Design review of the part built by this model. Coordinates are the model's own, in mm. A direction names the side the tool comes from. Coordinates: 2 decimals unless noted, no trailing zeros. Loops run counter-clockwise (first coordinate to the right, second up) from the corner with the lowest first, then second, coordinate; pieces in that order, holes last. Notation, with made-up numbers: (28, 26.25) -> (63, 26.25) arc R18 ccw to (63, 43.25) -> close; hole circle Ø3 at (39.25, -2.75). An arc over 180 degrees is marked (long way). Use a Markdown table: item, result. Add a question column.
Q1. Take a section at B-B on y = 20. Write out the cut boundary in (x, z), plus the area to 3 significant figures.
Q2. For faces 4 (the face through (-5.37, 0.99, 1.19)), 5 (the face through (7.3, -20, 0)), 6 (the face through (0, 80, 0)), 7 (the face through (5.38, 28.68, -8.43)), 8 (the face through (10, 20, 4.6)), list the 3-axis set-ups (+Z, -Z, +X, -X, +Y, -Y) from which the entire face can be reached by the end or side of a thin tool; tool diameter is ignored.
Q3. Take a section at A-A on y = -6.5. Write out the cut boundary in (x, z), plus the area to 3 significant figures.
Q4. Draft analysis for pull direction Z (two halves, no side actions). For faces 1 (the face through (5.684, 70.103, -1.79)), 2 (the face through (0.8, 8, 10.2)), 3 (the face through (3.64, 70.07, -1.15)), state which applies: pulls with the +Z half, pulls with the -Z half, needs draft (parallel to the pull), parting line crosses it, or undercut.
Q5. For probe 1 along X at (y, z) = (1.55, 0); probe 2 along X at (y, z) = (47, -0.5); probe 3 along Z at (x, y) = (0, 44.5), list the stretches that pass through material, from the lowest coordinate up.
Q6. Clearance check with flat-ended pins moving along their axes: pin 1 Ø12 at (x, z) = (0, 0) entering from -Y; pin 2 Ø10 at (x, y) = (7, 36.5) entering from +Z; pin 3 Ø3.5 at (x, z) = (4.5, 10) entering from +Y. State where each tip first meets the part, or that it passes through.
from build123d import *

# Parameters (mm, degrees)
SKETCH1_R               = 12
BOSS_EXTRUDE1_DEPTH     = 55
SKETCH2_R               = 2
SKETCH3_R               = 9
SKETCH3_R_2             = 7
BOSS_EXTRUDE2_DEPTH     = 20
SKETCH5_R               = 5.5
CUT_EXTRUDE2_DEPTH      = 4
SKETCH6_W               = 20
SKETCH6_H               = 25
CUT_EXTRUDE3_DEPTH      = 3
CUT_EXTRUDE4_DEPTH      = 85.380092576
CUT_EXTRUDE4_DEPTH_BACK = 85.380092576
SKETCH7_W               = 7.4
SKETCH7_H               = 25
FILLET1_R               = 1.5


# Read off the part's stored shape, not the designer's step: Shell1
with BuildPart() as part:
    # Sketch1 → Boss-Extrude1 (new body)
    with BuildSketch(Plane(origin=(0, 0, 0), x_dir=(1, 0, 0), z_dir=(0, 1, 0))):
        with Locations(Location((0, 0, 0), (0, 0, 270))):
            Circle(SKETCH1_R)
    extrude(amount=BOSS_EXTRUDE1_DEPTH)

    # Sketch2 → section 0 of loft1
    with BuildSketch(Plane(origin=(0, 80, 0), x_dir=(1, 0, 0), z_dir=(0, 1, 0)), mode=Mode.PRIVATE) as loft1_s0:
        Circle(SKETCH2_R)
    # loft up to a face of the part (loft1)
    loft([loft1_s0.sketch, Face(Wire([part.edges().sort_by_distance((8.747623529, 55, -8.214565271))[0]]))])

    # Shell1 outline → Shell1 (revolve, cut)
    with BuildSketch(Plane.XY):
        Polygon((10, 2), (10, 54.614835193), (0, 79.614835193), (0, 2), align=None)
    revolve(axis=Axis((0, 0, 0), (0, 1, 0)), mode=Mode.SUBTRACT)

    # Sketch3 → Boss-Extrude2 (add)
    with BuildSketch(Plane.XZ):
        with Locations(Location((0, 0, 0), (0, 0, 90))):
            Circle(SKETCH3_R)
        with Locations(Location((0, 0, 0), (0, 0, 270))):
            Circle(SKETCH3_R_2, mode=Mode.SUBTRACT)
    extrude(amount=BOSS_EXTRUDE2_DEPTH)

    # Sketch5 → Cut-Extrude2 (cut)
    with BuildSketch(Plane.XZ):
        with Locations(Location((0, 0, 0), (0, 0, 270))):
            Circle(SKETCH5_R)
    extrude(amount=-CUT_EXTRUDE2_DEPTH, mode=Mode.SUBTRACT)

    # Sketch6 → Cut-Extrude3 (cut, symmetric)
    with BuildSketch(Plane.XY.offset(11)):
        with Locations((0, 20.5)):
            Rectangle(SKETCH6_W, SKETCH6_H)
    extrude(amount=CUT_EXTRUDE3_DEPTH, both=True, mode=Mode.SUBTRACT)

    # Sketch7 → Cut-Extrude4 (cut, two sides: drawn at the far end of the back side and taken through both)
    with BuildSketch(Plane(origin=(-12, 0, 0), x_dir=(0, 0, -1), z_dir=(1, 0, 0)).offset(-CUT_EXTRUDE4_DEPTH_BACK)):
        with Locations((-8.3, 20.5)):
            Rectangle(SKETCH7_W, SKETCH7_H)
    extrude(amount=CUT_EXTRUDE4_DEPTH + CUT_EXTRUDE4_DEPTH_BACK, mode=Mode.SUBTRACT)

    # Fillet1
    fillet1_edges = [part.edges().sort_by_distance(p)[0] for p in [
        (0, 0, -9),
        (0, 0, -12),
    ]]
    fillet(fillet1_edges, radius=FILLET1_R - 0.0001)  # a hair under: the kernel refuses the full size


solid = part.part
Answer list:
| question | item | result |
|---|---|---|
| 1 | outline | (-11.08, 4.6) arc R12 ccw (long way) to (11.08, 4.6) -> (8.88, 4.6) arc R10 cw (long way) to (-8.88, 4.6) -> close |
| 1 | area | 88.1 mm² |
| 2 | face 4 | -Y |
| 2 | face 5 | +Z, -Z, +X, -X, -Y |
| 2 | face 6 | +Z, -Z, +X, -X, +Y |
| 2 | face 7 | none |
| 2 | face 8 | +Z, +X, -X |
| 3 | outline | circle Ø18 at (0, 0); hole circle Ø14 at (0, 0) |
| 3 | area | 101 mm² |
| 4 | face 1 | parting line crosses it |
| 4 | face 2 | needs draft |
| 4 | face 3 | undercut |
| 5 | probe 1 | -12 to -5.5, 5.5 to 12 |
| 5 | probe 2 | -11.99 to -9.99, 9.99 to 11.99 |
| 5 | probe 3 | -12 to -10, 10 to 12 |
| 6 | pin 1 | y = 0 |
| 6 | pin 2 | z = 11.83 |
| 6 | pin 3 | y = 61.96 |
